```python
from build123d import *

# Parameters (mm, degrees)
SKETCH1_W           = 38.1
SKETCH1_H           = 63.5
SKETCH1_W_2         = 31.75
SKETCH1_H_2         = 57.15
BOSS_EXTRUDE1_DEPTH = 76.2
SKETCH2_R           = 3.175
SKETCH2_W           = 38.1
SKETCH2_H           = 12.7
SKETCH2_R_2         = 4.7625
SKETCH2_R_3         = 3.96875
CUT_EXTRUDE1_DEPTH  = 39.1
CUT_EXTRUDE2_REACH  = 65.5
SKETCH3_W           = 31.75
SKETCH3_H           = 31.75
SKETCH3_H_2         = 22.225
CUT_EXTRUDE3_REACH  = 65.5
SKETCH4_W           = 31.75
SKETCH4_H           = 31.75
SKETCH4_H_2         = 25.4
FILLET1_R           = 3.175


with BuildPart() as part:
    # Sketch1 → Boss-Extrude1 (new body)
    with BuildSketch(Plane.XY):
        Rectangle(SKETCH1_W, SKETCH1_H)
        Rectangle(SKETCH1_W_2, SKETCH1_H_2, mode=Mode.SUBTRACT)
    extrude(amount=BOSS_EXTRUDE1_DEPTH)

    # Sketch2 → Cut-Extrude1 (cut, through all)
    with BuildSketch(Plane(origin=(19.05, 0, 0), x_dir=(0, 0, -1), z_dir=(1, 0, 0))):
        with Locations((-33.3375, -1.5875)):
            Circle(SKETCH2_R)
        with Locations((-68.2625, -1.5875)):
            Circle(SKETCH2_R)
        with Locations((-68.2625, -11.1125)):
            Circle(SKETCH2_R)
        with Locations((-33.3375, -11.1125)):
            Circle(SKETCH2_R)
        with Locations((-50.8, -6.35)):
            Rectangle(SKETCH2_W, SKETCH2_H)
        with BuildLine():
            ThreePointArc((-65.512869343, 0), (-70.50756403, 0.65756403), (-69.85, -4.337130657))
            Line((-69.85, -4.337130657), (-69.85, 0))
            Line((-69.85, 0), (-65.512869343, 0))
        make_face()
        with BuildLine():
            Line((-69.85, 0), (-69.85, -4.337130657))
            ThreePointArc((-69.85, -4.337130657), (-66.675, -4.337130657), (-65.0875, -1.5875))
            ThreePointArc((-65.0875, -1.5875), (-65.195685502, -0.765749532), (-65.512869343, 0))
            Line((-65.512869343, 0), (-69.85, 0))
        make_face()
        with BuildLine():
            ThreePointArc((-36.087130657, 0), (-35.58256403, -3.83256403), (-31.75, -4.337130657))
            Line((-31.75, -4.337130657), (-31.75, 0))
            Line((-31.75, 0), (-36.087130657, 0))
        make_face()
        with BuildLine():
            Line((-31.75, 0), (-31.75, -4.337130657))
            ThreePointArc((-31.75, -4.337130657), (-30.587869343, -3.175), (-30.1625, -1.5875))
            ThreePointArc((-30.1625, -1.5875), (-32.515749532, 1.479314498), (-36.087130657, 0))
            Line((-36.087130657, 0), (-31.75, 0))
        make_face()
        with BuildLine():
            ThreePointArc((-31.75, -8.362869343), (-35.58256403, -8.86743597), (-36.087130657, -12.7))
            Line((-36.087130657, -12.7), (-31.75, -12.7))
            Line((-31.75, -12.7), (-31.75, -8.362869343))
        make_face()
        with BuildLine():
            Line((-31.75, -12.7), (-36.087130657, -12.7))
            ThreePointArc((-36.087130657, -12.7), (-32.515749532, -14.179314498), (-30.1625, -11.1125))
            ThreePointArc((-30.1625, -11.1125), (-30.587869343, -9.525), (-31.75, -8.362869343))
            Line((-31.75, -8.362869343), (-31.75, -12.7))
        make_face()
        with BuildLine():
            Line((-69.85, -8.362869343), (-69.85, -12.7))
            Line((-69.85, -12.7), (-65.512869343, -12.7))
            ThreePointArc((-65.512869343, -12.7), (-65.195685502, -11.934250468), (-65.0875, -11.1125))
            ThreePointArc((-65.0875, -11.1125), (-66.675, -8.362869343), (-69.85, -8.362869343))
        make_face()
        with BuildLine():
            Line((-65.512869343, -12.7), (-69.85, -12.7))
            Line((-69.85, -12.7), (-69.85, -8.362869343))
            ThreePointArc((-69.85, -8.362869343), (-70.50756403, -13.35756403), (-65.512869343, -12.7))
        make_face()
        with Locations((-63.5, 15.875)):
            Circle(SKETCH2_R_2)
        with Locations((-12.7, -19.05)):
            Circle(SKETCH2_R_3)
    extrude(amount=-CUT_EXTRUDE1_DEPTH, mode=Mode.SUBTRACT)

    # Sketch3 → Cut-Extrude2 (cut, up to next)
    with BuildSketch(Plane(origin=(0, 31.75, 0), x_dir=(1, 0, 0), z_dir=(0, 1, 0)), mode=Mode.PRIVATE) as cut_extrude2_sk1:
        with Locations((0, -60.325)):
            Rectangle(SKETCH3_W, SKETCH3_H)
    cut_extrude2_tool1 = extrude(cut_extrude2_sk1.sketch, amount=-CUT_EXTRUDE2_REACH, mode=Mode.PRIVATE) & part.part
    add(cut_extrude2_tool1.solids().sort_by_distance((0, 31.75, 60.325))[0], mode=Mode.SUBTRACT)
    # Sketch3 → Cut-Extrude2 (cut, up to next)
    with BuildSketch(Plane(origin=(0, 31.75, 0), x_dir=(1, 0, 0), z_dir=(0, 1, 0)), mode=Mode.PRIVATE) as cut_extrude2_sk2:
        with Locations((0, -11.1125)):
            Rectangle(SKETCH3_W, SKETCH3_H_2)
    cut_extrude2_tool2 = extrude(cut_extrude2_sk2.sketch, amount=-CUT_EXTRUDE2_REACH, mode=Mode.PRIVATE) & part.part
    add(cut_extrude2_tool2.solids().sort_by_distance((0, 31.75, 11.1125))[0], mode=Mode.SUBTRACT)

    # Sketch4 → Cut-Extrude3 (cut, up to next)
    with BuildSketch(Plane.XZ.offset(31.75), mode=Mode.PRIVATE) as cut_extrude3_sk1:
        with Locations((0, 15.875)):
            Rectangle(SKETCH4_W, SKETCH4_H)
    cut_extrude3_tool1 = extrude(cut_extrude3_sk1.sketch, amount=-CUT_EXTRUDE3_REACH, mode=Mode.PRIVATE) & part.part
    add(cut_extrude3_tool1.solids().sort_by_distance((0, -31.75, 15.875))[0], mode=Mode.SUBTRACT)
    # Sketch4 → Cut-Extrude3 (cut, up to next)
    with BuildSketch(Plane.XZ.offset(31.75), mode=Mode.PRIVATE) as cut_extrude3_sk2:
        with Locations((0, 63.5)):
            Rectangle(SKETCH4_W, SKETCH4_H_2)
    cut_extrude3_tool2 = extrude(cut_extrude3_sk2.sketch, amount=-CUT_EXTRUDE3_REACH, mode=Mode.PRIVATE) & part.part
    add(cut_extrude3_tool2.solids().sort_by_distance((0, -31.75, 63.5))[0], mode=Mode.SUBTRACT)

    # Fillet1
    fillet1_edges = [part.edges().sort_by_distance(p)[0] for p in [
        (15.875, 30.1625, 44.45),
        (-15.875, 30.1625, 44.45),
        (15.875, 30.1625, 22.225),
        (-15.875, 30.1625, 22.225),
        (-15.875, -30.1625, 31.75),
        (15.875, -30.1625, 31.75),
        (-15.875, -30.1625, 50.8),
        (15.875, -30.1625, 50.8),
    ]]
    fillet(fillet1_edges, radius=FILLET1_R)


solid = part.part
```
Model file for the job. Use its own axes, mm. A direction names the side the tool comes from. Coordinates: 2 decimals unless noted, no trailing zeros. Loops run counter-clockwise (first coordinate to the right, second up) from the corner with the lowest first, then second, coordinate; pieces in that order, holes last. Notation, with made-up numbers: (12.25, 2) - (66.25, 2) arc R27 cw to (66.25, 20) - close; hole circle Ø4 at (-39.75, 77). An arc over 180 degrees is marked (long way). Answer as a JSON object with one key per item and string values. Group by question number.
(1) Cut at A-A (x = 1). Give the cut face in (y, z) (3 decimals), then the cut area to 3 significant figures.
(2) Two-plate mould, pull along Z, no slides. Class faces 1 (the face through (0, -30, 31.75)), 2 (the face through (0, -31.75, 38)), 3 (the face through (-17.44, -15.7, 10.57)): released by +Z, released by -Z, zero draft, split by the parting line, or undercut.
(3) Flat gauge pins, fed straight in: pin 1 (1.5 mm diameter, centred on x = 12.5, z = 53, fed in from -Y); pin 2 (1 mm diameter, centred on x = -0.5, y = -29.5, fed in from +Z). Where does each tip first touch, or does it go through?
(4) Probe line 1 along X through (y, z) = (17, 38) (3 decimals); line 2 along Y through (x, z) = (14.5, 32) (3 decimals); line 3 along Y through (x, z) = (17, 49). List the from-to ranges inside material, lowest first.
(5) Cut at D-D (z = 12.7). Give the cut face in (x, y) (3 decimals), then the cut area to 3 significant figures.
(6) Cut at B-B (y = -19.05). Give the cut face in (x, z) (3 decimals), then the cut area to 3 significant figures.
(7) Tool access for faces 4 (the face through (0, 30, 22.225)), 5 (the face through (14.92, -30.14, 30.845)), 6 (the face through (-14.97, -30.14, 51.755)), 7 (the face through (-17, -6, 69.85)), 8 (the face through (0, 31.75, 38)): list every direction of +Z, -Z, +X, -X, +Y, -Y with a clear straight run to the whole face (end or side of a thin tool).
(8) Cut at C-C (y = 4). Give the cut face in (x, z) (3 decimals).
Geometry says:
{
 "1": {"outline": "(-31.75, 31.75) - (-28.575, 31.75) - (-28.575, 50.8) - (-31.75, 50.8) - close; (28.575, 22.225) - (31.75, 22.225) - (31.75, 44.45) - (28.575, 44.45) - close", "area": "131 mm^2"},
 "2": {"face 1": "released by -Z", "face 2": "zero draft", "face 3": "undercut"},
 "3": {"pin 1": "passes through", "pin 2": "stops at z = 50.8"},
 "4": {"line 1": "x = -19.05 to -15.875, 15.875 to 19.05", "line 2": "y = -31.75 to -28.575, 28.575 to 31.75", "line 3": "y = -31.75 to -12.7, 0 to 31.75"},
 "5": {"outline": "(-19.05, -31.75) - (-15.875, -31.75) - (-15.875, -23.019) - (-19.05, -23.019) - close; (-19.05, -15.081) - (-15.875, -15.081) - (-15.875, 31.75) - (-19.05, 31.75) - close; (15.875, -31.75) - (19.05, -31.75) - (19.05, -23.019) - (15.875, -23.019) - close; (15.875, -15.081) - (19.05, -15.081) - (19.05, 31.75) - (15.875, 31.75) - close", "area": "353 mm^2"},
 "6": {"outline": "(-19.05, 0) - (-15.875, 0) - (-15.875, 8.731) - (-19.05, 8.731) - close; (-19.05, 16.669) - (-15.875, 16.669) - (-15.875, 76.2) - (-19.05, 76.2) - close; (15.875, 0) - (19.05, 0) - (19.05, 8.731) - (15.875, 8.731) - close; (15.875, 16.669) - (19.05, 16.669) - (19.05, 76.2) - (15.875, 76.2) - close", "area": "433 mm^2"},
 "7": {"face 4": "-Z, +Y, -Y", "face 5": "-Z, -Y", "face 6": "+Z, +Y, -Y", "face 7": "+X, -X", "face 8": "+Z, -Z, +X, -X, +Y"},
 "8": {"outline": "(-19.05, 0) - (-15.875, 0) - (-15.875, 76.2) - (-19.05, 76.2) - close; (15.875, 0) - (19.05, 0) - (19.05, 76.2) - (15.875, 76.2) - close"}
}
